Here's the drawing with two shaded views (mm, measured from the low corner). I have some questions. Coordinates: 2 decimals unless noted, no trailing zeros. Write each loop counter-clockwise with the first axis right and the second up, starting at its lowest first coordinate (ties: lowest second). Pieces come first, ordered by that corner, then holes.
Item 1: I want a section at B-B on y = 2.2. State how many separate pieces and enclosed holes the cut face has, then the cut area to 3 significant figures.
Item 2: I want a section at A-A on x = 273.05. Please give me the cut outline in (y, z).
Item 3: I want a section at C-C on z = 30.5. Please give me the cut outline in (x, y) (1 decimal).
Item 4: For P1, Ø5, axis at x = 273.05, z = 123.825, coming from the +Y side, with a flat end and sliding along its axis, tell me the tip position at first contact or that it passes through.
Item 5: I want a section at D-D on x = 139.7. Please give me the cut outline in (y, z).
Item 6: If I drill on probe 1 along Z at (x, y) = (273.05, 0.95); probe 2 along X at (y, z) = (2.25, 11); probe 3 along X at (y, z) = (0.8, 24), over which ranges is the centre line in solid material (lowest first)?
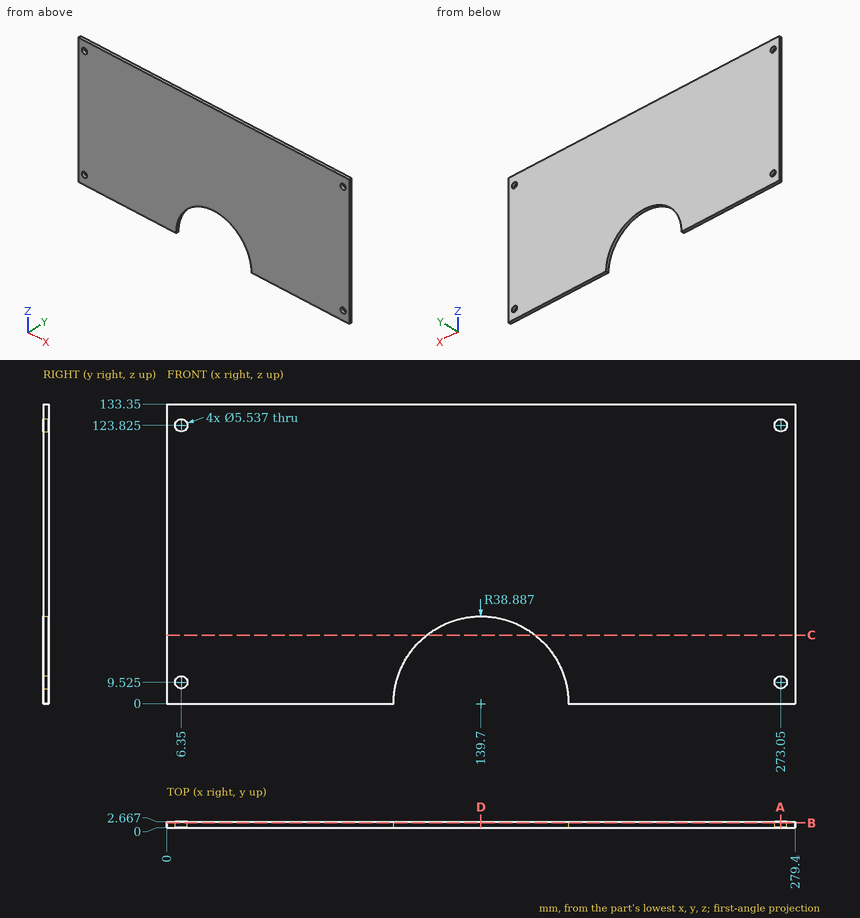
Response values:
1. separate pieces: 1
1. enclosed holes: 4
1. area: 34,800 mm2
2. outline: (0, 0) - (2.67, 0) - (2.67, 6.76) - (0, 6.76) - close; (0, 12.29) - (2.67, 12.29) - (2.67, 121.06) - (0, 121.06) - close; (0, 126.59) - (2.67, 126.59) - (2.67, 133.35) - (0, 133.35) - close
3. outline: (0, 0) - (115.6, 0) - (115.6, 2.7) - (0, 2.7) - close; (163.8, 0) - (279.4, 0) - (279.4, 2.7) - (163.8, 2.7) - close
4. P1: passes through
5. outline: (0, 38.89) - (2.67, 38.89) - (2.67, 133.35) - (0, 133.35) - close
6. probe 1: z = 0 to 6.76, 12.29 to 121.06, 126.59 to 133.35
6. probe 2: x = 0 to 4.01, 8.69 to 102.4, 177 to 270.71, 275.39 to 279.4
6. probe 3: x = 0 to 109.1, 170.3 to 279.4
